Geometry: final body of the model. Coordinates: model frame, mm. A direction names the side the tool comes from. Give positions to 0.01 mm unless a question says otherwise; leave off trailing zeros. Write each loop counter-clockwise with the first axis right and the second up, starting at its lowest first coordinate (ties: lowest second). Pieces come first, ordered by that corner, then holes. Notation, with made-up numbers: (15, -28.75) -> (57, -28.75) arc R37 ccw to (57, 8.25) -> close; hole circle Ø7 at (68, 67). An arc over 180 degrees is marked (long way). Answer as a JSON object with one key per item and string values. Group by question number.
(1) Section query D-D on y = 0.5. Output: boundary loops of the cut face in (x, z).
(2) Section query A-A on y = 20. Output: boundary loops of the cut face in (x, z), plus the area to 3 significant figures.
(3) Draft query along Y for faces 6 (the face through (-1, -30.5, 20)), 7 (the face through (-11, 18, 30)), 8 (the face through (1, 32.5, -1)). Return one class per face: +Y half, -Y half, draft (parallel to the pull), parting line (faces both ways), or undercut.
(4) Section query C-C on z = -2. Output: boundary loops of the cut face in (x, y), plus the area to 3 significant figures.
(5) Set-up query: faces 1 (the face through (-41, -13, 23)), 2 (the face through (-6, 15, -25)), 3 (the face through (7, -8, -28)), 4 (the face through (44, -29.5, -7)), 5 (the face through (0.644, -37.297, 28.859)). Return all of +Z, -Z, +X, -X, +Y, -Y with unobstructed straight access to the full face (end or side cutting, diameter ignored); none if empty.
(6) Contact query for flat-ended pins moving along their axis: pin 1 Ø1.5 at (x, z) = (13.5, 28.5) entering from -Y; pin 2 Ø3 at (y, z) = (0.5, -38) entering from +X; pin 3 Ø6.5 at (y, z) = (-23.5, -38) entering from +X; pin 4 Ø14.5 at (x, y) = (-19, 24) entering from -Z. Output: stop coordinate, or through.
(7) Section query B-B on x = -29. Output: boundary loops of the cut face in (y, z).
(8) Material intervals for probe 1 along Y at (x, z) = (4, -18); probe 2 along Y at (x, z) = (-37, -26); probe 3 along Y at (x, z) = (16, 15.5), sorted ascending.
from build123d import *

# Parameters (mm, degrees)
BASE_DEPTH               = 46
BASE_DEPTH_BACK          = 46
SKETCH4_W                = 60
SKETCH4_H                = 71
LIDAR_DEPTH              = 41
LIDAR_DEPTH_BACK         = 46
HOLEFRONTBACK_DEPTH      = 68.068994327
HOLEFRONTBACK_DEPTH_BACK = 68.068994327
SKETCH6_W                = 82
SKETCH6_H                = 45
FILLET2_R                = 4
BOSS_EXTRUDE1_DEPTH      = 4
BOSS_EXTRUDE1_DEPTH_BACK = 4
SKETCH11_W               = 18
SKETCH11_H               = 71
BOSS_EXTRUDE3_DEPTH      = 60
BOSS_EXTRUDE4_DEPTH      = 71
CUT_EXTRUDE1_START       = -57.309401
SKETCH14_R               = 2
CUT_EXTRUDE1_DEPTH       = 22.618802
CUT_EXTRUDE2_DEPTH       = 5
CHAMFER1_SIZE            = 4


with BuildPart() as part:
    # Sketch4 → Base (new, two sides: drawn at the far end of the back side and taken through both)
    with BuildSketch(Plane(origin=(0, 0, 0), x_dir=(0, 0, -1), z_dir=(1, 0, 0)).offset(-BASE_DEPTH_BACK)):
        with Locations((0, -3)):
            Rectangle(SKETCH4_W, SKETCH4_H)
    extrude(amount=BASE_DEPTH + BASE_DEPTH_BACK)

    # Sketch5 → LIDAR (cut, two sides: drawn at the far end of the back side and taken through both)
    with BuildSketch(Plane(origin=(0, 0, 0), x_dir=(0, 0, -1), z_dir=(1, 0, 0)).offset(-LIDAR_DEPTH_BACK)):
        Polygon((-25, 27.5), (-25, 14.5), (-10.630657971, -32.5), (25, -32.5), (25, 27.5), align=None)
    extrude(amount=LIDAR_DEPTH + LIDAR_DEPTH_BACK, mode=Mode.SUBTRACT)

    # Sketch6 → HoleFrontBack (cut, two sides: drawn at the far end of the back side and taken through both)
    with BuildSketch(Plane.XY.offset(-HOLEFRONTBACK_DEPTH_BACK)):
        with Locations((0, -8)):
            Rectangle(SKETCH6_W, SKETCH6_H)
    extrude(amount=HOLEFRONTBACK_DEPTH + HOLEFRONTBACK_DEPTH_BACK, mode=Mode.SUBTRACT)

    # Fillet2
    fillet2_edges = [part.edges().sort_by_distance(p)[0] for p in [
        (0, 32.5, 30),
        (0, 32.5, -30),
        (0, -38.5, -30),
        (0, -38.5, 30),
    ]]
    fillet(fillet2_edges, radius=FILLET2_R)

    # Sketch11 → Boss-Extrude1 (add, two sides: drawn at the far end of the back side and taken through both)
    with BuildSketch(Plane(origin=(0, 0, -30), x_dir=(-1, 0, 0), z_dir=(0, 0, -1)).offset(-BOSS_EXTRUDE1_DEPTH_BACK)):
        with Locations((0, -3)):
            Rectangle(SKETCH11_W, SKETCH11_H)
    extrude(amount=BOSS_EXTRUDE1_DEPTH + BOSS_EXTRUDE1_DEPTH_BACK)

    # Sketch13 → Boss-Extrude3 (add)
    with BuildSketch(Plane(origin=(0, 0, -34), x_dir=(-1, 0, 0), z_dir=(0, 0, -1))):
        Polygon((-9, -38.5), (9, -38.5), (11.309401077, -42.5), (9, -46.5), (-9, -46.5), (-11.309401077, -42.5), align=None)
    extrude(amount=-BOSS_EXTRUDE3_DEPTH)

    # Sketch12 → Boss-Extrude4 (add)
    with BuildSketch(Plane(origin=(0, 32.5, 0), x_dir=(1, 0, 0), z_dir=(0, 1, 0))):
        Polygon((-9, 34), (-11.309401077, 38), (-9, 42), (9, 42), (11.309401077, 38), (9, 34), align=None)
    extrude(amount=-BOSS_EXTRUDE4_DEPTH)

    # Sketch14 → Cut-Extrude1 (cut)
    with BuildSketch(Plane(origin=(46, 0, 0), x_dir=(0, 0, -1), z_dir=(1, 0, 0)).offset(CUT_EXTRUDE1_START)):
        with Locations(Location((38, 24.5, 0), (0, 0, 90))):
            Circle(SKETCH14_R)
        with Locations(Location((38, 16.5, 0), (0, 0, 90))):
            Circle(SKETCH14_R)
        with Locations(Location((38, 8.5, 0), (0, 0, 90))):
            Circle(SKETCH14_R)
        with Locations(Location((38, 0.5, 0), (0, 0, 90))):
            Circle(SKETCH14_R)
        with Locations(Location((38, -7.5, 0), (0, 0, 90))):
            Circle(SKETCH14_R)
        with Locations(Location((38, -15.5, 0), (0, 0, 90))):
            Circle(SKETCH14_R)
        with Locations(Location((38, -23.5, 0), (0, 0, 90))):
            Circle(SKETCH14_R)
        with Locations(Location((38, -31.5, 0), (0, 0, 90))):
            Circle(SKETCH14_R)
        with Locations((26, -42.5)):
            Circle(SKETCH14_R)
        with Locations((18, -42.5)):
            Circle(SKETCH14_R)
        with Locations((10, -42.5)):
            Circle(SKETCH14_R)
        with Locations((2, -42.5)):
            Circle(SKETCH14_R)
        with Locations((-6, -42.5)):
            Circle(SKETCH14_R)
        with Locations((-14, -42.5)):
            Circle(SKETCH14_R)
        with Locations((-22, -42.5)):
            Circle(SKETCH14_R)
    extrude(amount=CUT_EXTRUDE1_DEPTH, mode=Mode.SUBTRACT)

    # Sketch15 → Cut-Extrude2 (cut)
    with BuildSketch(Plane(origin=(46, 0, 0), x_dir=(0, 0, -1), z_dir=(1, 0, 0))):
        Polygon((-22, 14.948353004), (-8.410774746, -29.5), (22, -29.5), (22, 14.641172912), (22, 24.5), (-22, 24.5), align=None)
    extrude(amount=-CUT_EXTRUDE2_DEPTH, mode=Mode.SUBTRACT)

    # Chamfer1
    chamfer1_edges = [part.edges().sort_by_distance(p)[0] for p in [
        (9, -8, -26),
        (-9, -8, -26),
    ]]
    chamfer(chamfer1_edges, length=CHAMFER1_SIZE)


solid = part.part
Answer list:
{
 "1": {"outline": "(-46, -30) -> (-41, -30) -> (-41, -25) -> (-46, -25) -> close; (-46, 20.72) -> (-41, 20.72) -> (-41, 30) -> (-46, 30) -> close; (-10.15, -40) -> (-9, -42) -> (9, -42) -> (10.15, -40) -> close; (-10.15, -36) -> (10.15, -36) -> (9, -34) -> (9, -30) -> (5, -26) -> (-5, -26) -> (-9, -30) -> (-9, -34) -> close; (41, -30) -> (46, -30) -> (46, -22) -> (41, -22) -> close; (41, 17.58) -> (46, 17.58) -> (46, 30) -> (41, 30) -> close"},
 "2": {"outline": "(-46, -30) -> (-9, -30) -> (-9, -34) -> (-11.31, -38) -> (-9, -42) -> (9, -42) -> (11.31, -38) -> (9, -34) -> (9, -30) -> (46, -30) -> (46, -22) -> (41, -22) -> (41, -25) -> (-46, -25) -> close; (-46, 25) -> (41, 25) -> (41, 22) -> (46, 22) -> (46, 30) -> (-46, 30) -> close", "area": "1,180 mm2"},
 "3": {"face 6": "undercut", "face 7": "draft", "face 8": "+Y half"},
 "4": {"outline": "(-46, -38.5) -> (-9, -38.5) -> (-10.15, -40.5) -> (10.15, -40.5) -> (9, -38.5) -> (46, -38.5) -> (46, -29.5) -> (41, -29.5) -> (41, -32.5) -> (-46, -32.5) -> close; (-46, 27.5) -> (41, 27.5) -> (41, 24.5) -> (46, 24.5) -> (46, 32.5) -> (-46, 32.5) -> close; (-10.15, -44.5) -> (-9, -46.5) -> (9, -46.5) -> (10.15, -44.5) -> close", "area": "1,120 mm2"},
 "5": {"face 1": "+Z, -Z", "face 2": "-X", "face 3": "+Z", "face 4": "+X, -X", "face 5": "+Z, +X, -X, -Y"},
 "6": {"pin 1": "y = -38.1", "pin 2": "through", "pin 3": "x = 11.31", "pin 4": "z = -30"},
 "7": {"outline": "(-38.5, -26) arc R4 ccw to (-34.5, -30) -> (-30.5, -30) -> (-30.5, -25) -> (-32.5, -25) -> (-32.5, 10.63) -> (-30.5, 11.24) -> (-30.5, 30) -> (-34.5, 30) arc R4 ccw to (-38.5, 26) -> close; (14.5, -30) -> (28.5, -30) arc R4 ccw to (32.5, -26) -> (32.5, 26) arc R4 ccw to (28.5, 30) -> (14.5, 30) -> (14.5, 25) -> (27.5, 25) -> (27.5, -25) -> (14.5, -25) -> close"},
 "8": {"probe 1": "-46.5 to -44.5, -40.5 to -32.5, 27.5 to 32.5", "probe 2": "-38.5 to -30.5, 14.5 to 32.5", "probe 3": "-38.5 to -30.5, 27.5 to 32.5"}
}
